Geometry check sheet. Reference: the model listing, model coordinates, mm. A direction names the side the tool comes from. Round coordinates to 2 decimals unless told otherwise and drop trailing zeros. Loops run counter-clockwise (first coordinate to the right, second up) from the corner with the lowest first, then second, coordinate; pieces in that order, holes last. Notation, with made-up numbers: (-32, -24.5) -> (-14, -24.5) arc R24 cw to (-14, 1.5) -> close; hole circle Ø2 at (-26, 13). An arc over 180 degrees is marked (long way). Use one line per item in the form item = value.
from build123d import *

# Parameters (mm, degrees)
SKETCH1_W           = 66
SKETCH1_H           = 68
SKETCH1_R           = 1
SKETCH1_W_2         = 17.8
SKETCH1_H_2         = 7.6
BOSS_EXTRUDE1_DEPTH = 2


with BuildPart() as part:
    # Sketch1 → Boss-Extrude1 (new body)
    with BuildSketch(Plane.XY.offset(30)):
        with Locations((251.940861289, 301.024014524)):
            Rectangle(SKETCH1_W, SKETCH1_H)
        with Locations((249.003592831, 330.031505481)):
            Circle(SKETCH1_R, mode=Mode.SUBTRACT)
        with Locations((255.055282531, 330.031505481)):
            Circle(SKETCH1_R, mode=Mode.SUBTRACT)
        with Locations((252.135035756, 320.823888471)):
            Rectangle(SKETCH1_W_2, SKETCH1_H_2, mode=Mode.SUBTRACT)
    extrude(amount=BOSS_EXTRUDE1_DEPTH)


solid = part.part
1. Tool access check on faces 1 (the flat face through (251, 335.024, 31)), 2 (the flat face through (243.235, 321, 31)). Record the directions out of +Z, -Z, +X, -X, +Y, -Y that give a thin tool (end or side, any length) a straight path to the whole face; none if there is none.
Return value:
face_1 = +Z, -Z, +X, -X, +Y
face_2 = +Z, -Z
2. Section check B-B (z = 31.45). Record the boundary of the cut face in (x, y).
Return value:
outline = (218.94, 267.02) -> (284.94, 267.02) -> (284.94, 335.02) -> (218.94, 335.02) -> close; hole (243.24, 317.02) -> (261.04, 317.02) -> (261.04, 324.62) -> (243.24, 324.62) -> close; hole circle Ø2 at (249, 330.03); hole circle Ø2 at (255.06, 330.03)
3. Gauge pin test, flat end, axial feed: pin 1 (1.8 mm diameter, centred on x = 255.06, y = 330.03, fed in from -Z). Record the tip position at first contact, or that the pin passes through.
Return value:
pin_1 = through
4. Material ranges on line 1 along X through (y, z) = (330, 31.1); line 2 along Y through (x, z) = (261, 31.95); line 3 along Y through (x, z) = (255, 31.85), recorded low to high.
Return value:
line_1 = 218.94 to 248, 250 to 254.06, 256.05 to 284.94
line_2 = 267.02 to 317.02, 324.62 to 335.02
line_3 = 267.02 to 317.02, 324.62 to 329.03, 331.03 to 335.02
5. Mould release check, pull along Y, two halves, no side actions. Record for faces 3 (the flat face through (251, 267.024, 31)), 4 (the flat face through (251, 302, 30)), 5 (the flat face through (252, 324.624, 31)), 6 (the cylindrical face through (248.21, 329.42, 30.99)): released by +Y, released by -Y, zero draft, split by the parting line, or undercut.
Return value:
face_3 = released by -Y
face_4 = zero draft
face_5 = undercut
face_6 = undercut
6. Section check A-A (x = 245.5). Record the boundary of the cut face in (y, z), then the cut area to 3 significant figures.
Return value:
outline = (267.02, 30) -> (317.02, 30) -> (317.02, 32) -> (267.02, 32) -> close; (324.62, 30) -> (335.02, 30) -> (335.02, 32) -> (324.62, 32) -> close
area = 121 mm2
